Input: part model. Units: mm. Frame: model coordinates. A direction names the side the tool comes from. Round coordinates to 2 decimals unless told otherwise and drop trailing zeros. Order: outer loops, then holes, each group sorted by start corner. A loop starts at its lowest first (then second) coordinate and runs counter-clockwise, first axis right, second up. Notation, with made-up numbers: (26.25, -10.75) -> (48.25, -10.75) arc R24 ccw to (48.25, 8.25) -> close; hole circle Ø9 at (-26, -9). An arc over 180 degrees is marked (long way). Use a Markdown table: item, result.
from build123d import *

# Parameters (mm, degrees)
IZIM1_R                     = 195
IZIM1_R_2                   = 185
Y_KSEKLIK_EKSTR_ZYON1_DEPTH = 10
KES_EKSTR_ZYON1_DEPTH       = 250
KES_EKSTR_ZYON1_DEPTH_BACK  = 240
IZIM2_R                     = 1
KES_EKSTR_ZYON2_DEPTH       = 240
KES_EKSTR_ZYON2_DEPTH_BACK  = 240
IZIM3_R                     = 1
KES_EKSTR_ZYON3_DEPTH       = 139
IZIM6_W                     = 5
IZIM6_H                     = 10
Y_KSEKLIK_EKSTR_ZYON2_DEPTH = 8
IZIM7_W                     = 5
IZIM7_H                     = 10
Y_KSEKLIK_EKSTR_ZYON3_DEPTH = 8


with BuildPart() as part:
    # izim1 → Y_kseklik-Ekstr_zyon1 (new body)
    with BuildSketch(Plane.XY):
        Circle(IZIM1_R)
        Circle(IZIM1_R_2, mode=Mode.SUBTRACT)
    extrude(amount=Y_KSEKLIK_EKSTR_ZYON1_DEPTH)

    # izim2 → Kes-Ekstr_zyon1 (cut, two sides: drawn at the far end of the back side and taken through both)
    with BuildSketch(Plane(origin=(0, 0, 0), x_dir=(0, 0, -1), z_dir=(1, 0, 0)).offset(-KES_EKSTR_ZYON1_DEPTH_BACK)):
        with Locations(Location((-5, 0, 0), (0, 0, 180))):
            Circle(IZIM2_R)
    extrude(amount=KES_EKSTR_ZYON1_DEPTH + KES_EKSTR_ZYON1_DEPTH_BACK, mode=Mode.SUBTRACT)

    # izim3 → Kes-Ekstr_zyon2 (cut, two sides: drawn at the far end of the back side and taken through both)
    with BuildSketch(Plane(origin=(0, 0, 0), x_dir=(1, 0, 0), z_dir=(0, 1, 0)).offset(-KES_EKSTR_ZYON2_DEPTH_BACK)):
        with Locations(Location((0, -5, 0), (0, 0, 90))):
            Circle(IZIM3_R)
    extrude(amount=KES_EKSTR_ZYON2_DEPTH + KES_EKSTR_ZYON2_DEPTH_BACK, mode=Mode.SUBTRACT)

    # izim4 → Kes-Ekstr_zyon3 (cut)
    with BuildSketch(Plane(origin=(0, 0, 0), x_dir=(-1, 0, 0), z_dir=(0, 0, -1))):
        with BuildLine():
            ThreePointArc((-137.885822331, -137.885822331), (195, 0), (-137.885822331, 137.885822331))
            Line((-137.885822331, 137.885822331), (-130.81475452, 130.81475452))
            ThreePointArc((-130.81475452, 130.81475452), (185, 0), (-130.81475452, -130.81475452))
            Line((-130.81475452, -130.81475452), (-137.885822331, -137.885822331))
        make_face()
    extrude(amount=-KES_EKSTR_ZYON3_DEPTH, mode=Mode.SUBTRACT)

    # izim6 → Y_kseklik-Ekstr_zyon2 (add)
    with BuildSketch(Plane(origin=(0, 0, 0), x_dir=(0, 0, 1), z_dir=(-0.7071067811865477, -0.7071067811865475, 0))):
        with Locations((7.5, -190)):
            Rectangle(IZIM6_W, IZIM6_H)
    extrude(amount=Y_KSEKLIK_EKSTR_ZYON2_DEPTH)

    # izim7 → Y_kseklik-Ekstr_zyon3 (add)
    with BuildSketch(Plane(origin=(0, 0, 0), x_dir=(0, 0, 1), z_dir=(-0.7071067811865477, 0.7071067811865475, 0))):
        with Locations((2.5, 190)):
            Rectangle(IZIM7_W, IZIM7_H)
    extrude(amount=Y_KSEKLIK_EKSTR_ZYON3_DEPTH)


solid = part.part
1) Contact query for flat-ended pins moving along their axis: P1, Ø6, axis at y = 109, z = 8, coming from the +X side; P2, Ø6.5, axis at x = 131.5, y = -135.5, coming from the -Z side; P3, Ø5, axis at y = -50, z = 6, coming from the -X side; P4, Ø2, axis at y = -58, z = 7, coming from the +X side. Output: stop coordinate, or through.
Answer key:
| item | result |
|---|---|
| P1 | stops at x = 163.67 |
| P2 | stops at z = 0 |
| P3 | stops at x = 177.39 |
| P4 | stops at x = 186.48 |
2) Cut plane C-C on y = 124. Return loops of the section in (x, z).
Answer key:
| item | result |
|---|---|
| outline | (137.29, 0) -> (150.5, 0) -> (150.5, 10) -> (137.29, 10) -> close |
3) Set-up query: faces 1 (the face through (134, -134, 2)), 2 (the face through (128.03, -133.6, 7.46)), 3 (the face through (132, 137, 5)). Return all of +Z, -Z, +X, -X, +Y, -Y with unobstructed straight access to the full face (end or side cutting, diameter ignored); none if empty.
Answer key:
| item | result |
|---|---|
| face 1 | -Z, -X, -Y |
| face 2 | +Z, -Z, -X, +Y |
| face 3 | +Z, -X, +Y |
4) Cut plane B-B on x = 158.5. Return loops of the section in (y, z).
Answer key:
| item | result |
|---|---|
| outline | (-113.59, 0) -> (-95.41, 0) -> (-95.41, 10) -> (-113.59, 10) -> close; (95.41, 0) -> (113.59, 0) -> (113.59, 10) -> (95.41, 10) -> close |
5) Cut plane A-A on x = 176. Return loops of the section in (y, z), and give its area (3 significant figures).
Answer key:
| item | result |
|---|---|
| outline | (-83.96, 0) -> (-57, 0) -> (-57, 10) -> (-83.96, 10) -> close; (57, 0) -> (83.96, 0) -> (83.96, 10) -> (57, 10) -> close |
| area | 539 mm^2 |
6) Cut plane D-D on x = 135. Return loops of the section in (y, z).
Answer key:
| item | result |
|---|---|
| outline | (-140.77, 5) -> (-135, 5) -> (-135, 0) -> (-126.49, 0) -> (-126.49, 10) -> (-140.77, 10) -> close; (126.49, 0) -> (140.77, 0) -> (140.77, 5) -> (135, 5) -> (135, 10) -> (126.49, 10) -> close |
7) Ray query, probe 1 along Y at (x, z) = (165, 8.5); probe 2 along Y at (x, z) = (146.5, 8); probe 3 along X at (y, z) = (-60.5, 7). Return the intervals inside material, ascending.
Answer key:
| item | result |
|---|---|
| probe 1 | y = -103.92 to -83.67, 83.67 to 103.92 |
| probe 2 | y = -128.7 to -112.97, 112.97 to 128.7 |
| probe 3 | x = 174.83 to 185.38 |
8) Draft query along Y for faces 4 (the face through (188, -2, 10)), 5 (the face through (184.99, -2.03, 4.93)), 6 (the face through (135.1, -140.67, 7.46)). Return one class per face: released by +Y, released by -Y, zero draft, split by the parting line, or undercut.
Answer key:
| item | result |
|---|---|
| face 4 | zero draft |
| face 5 | undercut |
| face 6 | released by -Y |
